```python
from build123d import *

# Parameters (mm, degrees)
FILLET1_R = 5


with BuildPart() as part:
    # Sketch1 → Revolve3 (revolve)
    with BuildSketch(Plane.XY):
        with BuildLine():
            Line((-27.5, -13), (-27.5, -12))
            Line((-27.5, -12), (-24.9, -12))
            ThreePointArc((-24.9, -12), (-23.057568057, 0), (-24.9, 12))
            Line((-24.9, 12), (-27.5, 12))
            Line((-27.5, 12), (-27.5, 13))
            Line((-27.5, 13), (-37.5, 13))
            Line((-37.5, 13), (-37.5, -13))
            Line((-37.5, -13), (-27.5, -13))
        make_face()
    revolve(axis=Axis((0, 39.143904287, 0), (0, -1, 0)))

    # Fillet1
    fillet1_edges = [part.edges().sort_by_distance(p)[0] for p in [
        (37.5, -13, 0),
        (37.5, 13, 0),
    ]]
    fillet(fillet1_edges, radius=FILLET1_R)


solid = part.part
```
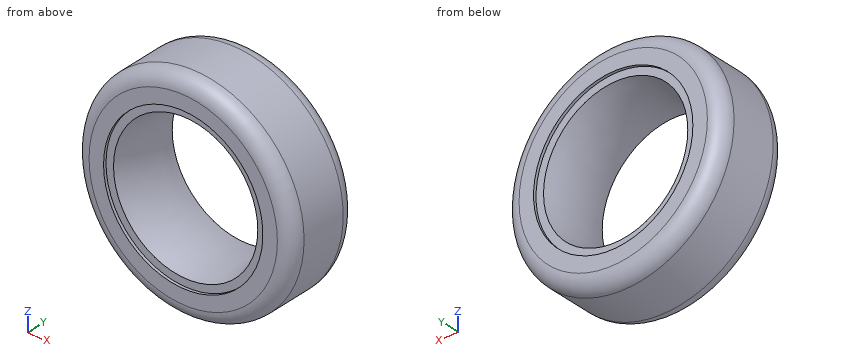
Geometry: final body of the model. Coordinates: model frame, mm. Round coordinates to 2 decimals unless told otherwise and drop trailing zeros. Order: outer loops, then holes, each group sorted by start corner. A loop starts at its lowest first (then second) coordinate and runs counter-clockwise, first axis right, second up. Notation, with made-up numbers: (54.5, 24.5) -> (66.5, 24.5) arc R23 cw to (66.5, 60.5) -> close; hole circle Ø5 at (10, 64). An arc over 180 degrees is marked (long way). Use one line per item in the form item = value. Start each with the question number.
1. Cut plane C-C (y = -0.5). Return the cut outline in (x, z), then the cut area to 3 significant figures.
2. Cut plane A-A (z = 0). Return the cut outline in (x, y), then the cut area to 3 significant figures.
3. Cut plane D-D (y = -4.5). Return the cut outline in (x, z).
4. Cut plane B-B (x = 0). Return the cut outline in (y, z), then the cut area to 3 significant figures.
5. Pin query (flat end, axial travel): pin 1 Ø1.5 at (y, z) = (3, 26.5) entering from -X; pin 2 Ø4 at (x, y) = (21, -4.5) entering from -Z; pin 3 Ø10 at (x, y) = (9, 4) entering from -Z. Return the tip coordinate at first contact, or that it passes through.
6. Line query: probe 1 along Y at (x, z) = (-26, -1.5); probe 2 along Z at (x, y) = (0, 12.2); probe 3 along X at (y, z) = (12.4, 0). Output: solid intervals per line, ascending.
Solution:
q1.outline = circle Ø75 at (0, 0); hole circle Ø46.12 at (0, 0)
q1.area = 2,750 mm^2
q2.outline = (-37.5, -8) arc R5 ccw to (-32.5, -13) -> (-27.5, -13) -> (-27.5, -12) -> (-24.9, -12) arc R40 ccw to (-24.9, 12) -> (-27.5, 12) -> (-27.5, 13) -> (-32.5, 13) arc R5 ccw to (-37.5, 8) -> close; (24.9, -12) -> (27.5, -12) -> (27.5, -13) -> (32.5, -13) arc R5 ccw to (37.5, -8) -> (37.5, 8) arc R5 ccw to (32.5, 13) -> (27.5, 13) -> (27.5, 12) -> (24.9, 12) arc R40 ccw to start
q2.area = 683 mm^2
q3.outline = circle Ø75 at (0, 0); hole circle Ø46.62 at (0, 0)
q4.outline = (-13, -32.5) arc R5 ccw to (-8, -37.5) -> (8, -37.5) arc R5 ccw to (13, -32.5) -> (13, -27.5) -> (12, -27.5) -> (12, -24.9) arc R40 ccw to (-12, -24.9) -> (-12, -27.5) -> (-13, -27.5) -> close; (-13, 27.5) -> (-12, 27.5) -> (-12, 24.9) arc R40 ccw to (12, 24.9) -> (12, 27.5) -> (13, 27.5) -> (13, 32.5) arc R5 ccw to (8, 37.5) -> (-8, 37.5) arc R5 ccw to (-13, 32.5) -> close
q4.area = 683 mm^2
q5.pin_1 = -27.26
q5.pin_2 = -32.33
q5.pin_3 = -37.29
q6.probe_1 = -12 to 12
q6.probe_2 = -35.21 to -27.5, 27.5 to 35.21
q6.probe_3 = -34.87 to -27.5, 27.5 to 34.87
